from build123d import *

# Parameters (mm, degrees)
ESBO_O1_R                = 7.5
RESSALTO_EXTRUS_O1_DEPTH = 100
ESBO_O2_W                = 5
ESBO_O2_H                = 45
RESSALTO_EXTRUS_O2_DEPTH = 9.5
CORTE_EXTRUS_O2_START    = -10
CORTE_EXTRUS_O2_DEPTH    = 10
CORTE_EXTRUS_O3_START    = -10
CORTE_EXTRUS_O3_DEPTH    = 10


with BuildPart() as part:
    # Esboço1 → Ressalto-extrusão1 (new body)
    with BuildSketch(Plane.XY):
        Circle(ESBO_O1_R)
    extrude(amount=-RESSALTO_EXTRUS_O1_DEPTH)

    # Esboço2 → Ressalto-extrusão2 (add)
    with BuildSketch(Plane(origin=(0, 0, 0), x_dir=(1, 0, 0), z_dir=(0, 1, 0))):
        with Locations((0, 28.25)):
            Rectangle(ESBO_O2_W, ESBO_O2_H)
    extrude(amount=RESSALTO_EXTRUS_O2_DEPTH)

    # Esboço3 → Corte-extrusão2 (cut)
    with BuildSketch(Plane(origin=(0, 0, -100), x_dir=(-1, 0, 0), z_dir=(0, 0, -1)).offset(CORTE_EXTRUS_O2_START)):
        with BuildLine():
            ThreePointArc((3.741657387, 6.5), (0, 7.5), (-3.741657387, 6.5))
            Line((-3.741657387, 6.5), (-3.242769735, 5.633333333))
            ThreePointArc((-3.242769735, 5.633333333), (0, 6.5), (3.242769735, 5.633333333))
            Line((3.242769735, 5.633333333), (3.741657387, 6.5))
        make_face()
    extrude(amount=CORTE_EXTRUS_O2_DEPTH, mode=Mode.SUBTRACT)

    # Esboço3<5> → Corte-extrusão3 (cut)
    with BuildSketch(Plane(origin=(0, 0, -100), x_dir=(-1, 0, 0), z_dir=(0, 0, -1)).offset(CORTE_EXTRUS_O3_START)):
        with BuildLine():
            Line((-6.5, 0), (-7.5, 0))
            ThreePointArc((-7.5, 0), (-6.492781777, -3.754168989), (-3.741657387, -6.5))
            Line((-3.741657387, -6.5), (-3.242769735, -5.633333333))
            ThreePointArc((-3.242769735, -5.633333333), (-5.62707754, -3.253613124), (-6.5, 0))
        make_face()
        with BuildLine():
            ThreePointArc((6.5, 0), (5.863181424, -2.805905129), (4.077506587, -5.062009485))
            Line((4.077506587, -5.062009485), (4.704815293, -5.840780175))
            ThreePointArc((4.704815293, -5.840780175), (6.765209335, -3.237582841), (7.5, 0))
            Line((7.5, 0), (6.5, 0))
        make_face()
    extrude(amount=CORTE_EXTRUS_O3_DEPTH, mode=Mode.SUBTRACT)


solid = part.part
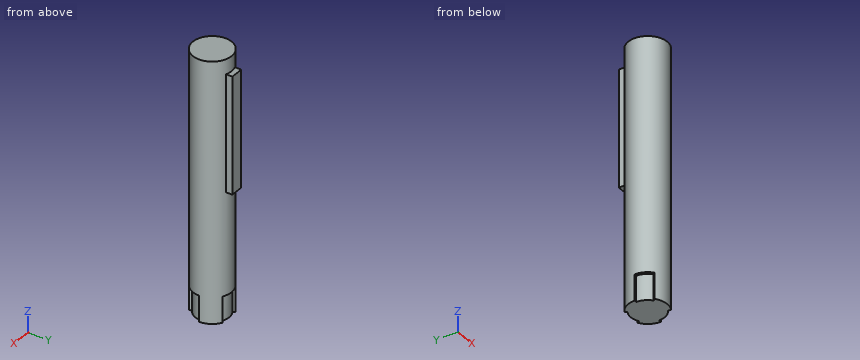
Design review of the part built by this model. Coordinates are the model's own, in mm. Coordinates: 2 decimals unless noted, no trailing zeros. Loops run counter-clockwise (first coordinate to the right, second up) from the corner with the lowest first, then second, coordinate; pieces in that order, holes last. Notation, with made-up numbers: M -11,2 L 6,2 A17 cw 6,34 Z; hole C -33,37.25 d4. An arc over 180 degrees is marked long. Answer as CSV lines item,"result".
Item 1: Add section A-A on x = 0. State the section outline as (y, z) points.
Answer list:
outline,"M -7.5,-100 L 6.5,-100 L 6.5,-90 L 7.5,-90 L 7.5,-50.75 L 9.5,-50.75 L 9.5,-5.75 L 7.5,-5.75 L 7.5,0 L -7.5,0 Z"
Item 2: For P1, Ø1.5, axis at y = -1.5, z = -41.5, coming from the +X side; P2, Ø2, axis at x = 5.5, y = -4.5, coming from the -Z side; P3, Ø1, axis at y = -1, z = -64, coming from the -X side; P4, Ø8, axis at y = -5, z = -88.5, coming from the +X side, all flat-tipped, find the tip position at first contact; note any pin that passes through.
Answer list:
P1,"x = 7.46"
P2,"z = -100"
P3,"x = -7.48"
P4,"x = 7.43"
Item 3: For probe 1 along Y at (x, z) = (-6.5, -21); probe 2 along Z at (x, y) = (-2.25, 6.75); probe 3 along X at (y, z) = (8.25, -50), list the stretches that pass through material, from the lowest coordinate up.
Answer list:
probe 1,"-3.74 to 3.74"
probe 2,"-90 to 0"
probe 3,"-2.5 to 2.5"
Item 4: Add section B-B on z = -77. State the section outline as (x, y) points.
Answer list:
outline,"C 0,0 d15"
Item 5: Add section C-C on y = -2.25. State the section outline as (x, z) points, plus the area to 3 significant figures.
Answer list:
outline,"M -7.15,-90 L -6.1,-90 L -6.1,-100 L 6.1,-100 L 6.1,-90 L 7.15,-90 L 7.15,0 L -7.15,0 Z"
area,"1,410 mm²"
Item 6: Add section D-D on z = -24.5. State the section outline as (x, y) points, plus the area to 3 significant figures.
Answer list:
outline,"M -2.5,7.07 A7.5 ccw long 2.5,7.07 L 2.5,9.5 L -2.5,9.5 Z"
area,"187 mm²"
